Part print with two shaded views. Sizes in mm from the minimum x, y, z corner. Round coordinates to 2 decimals unless told otherwise and drop trailing zeros. Loops run counter-clockwise (first coordinate to the right, second up) from the corner with the lowest first, then second, coordinate; pieces in that order, holes last. Notation, with made-up numbers: (47, -33) -> (105, -33) arc R10 ccw to (105, -27) -> close; hole circle Ø1 at (-39, -34.75). An arc over 180 degrees is marked (long way). Use a Markdown table: item, result. Add a question column.
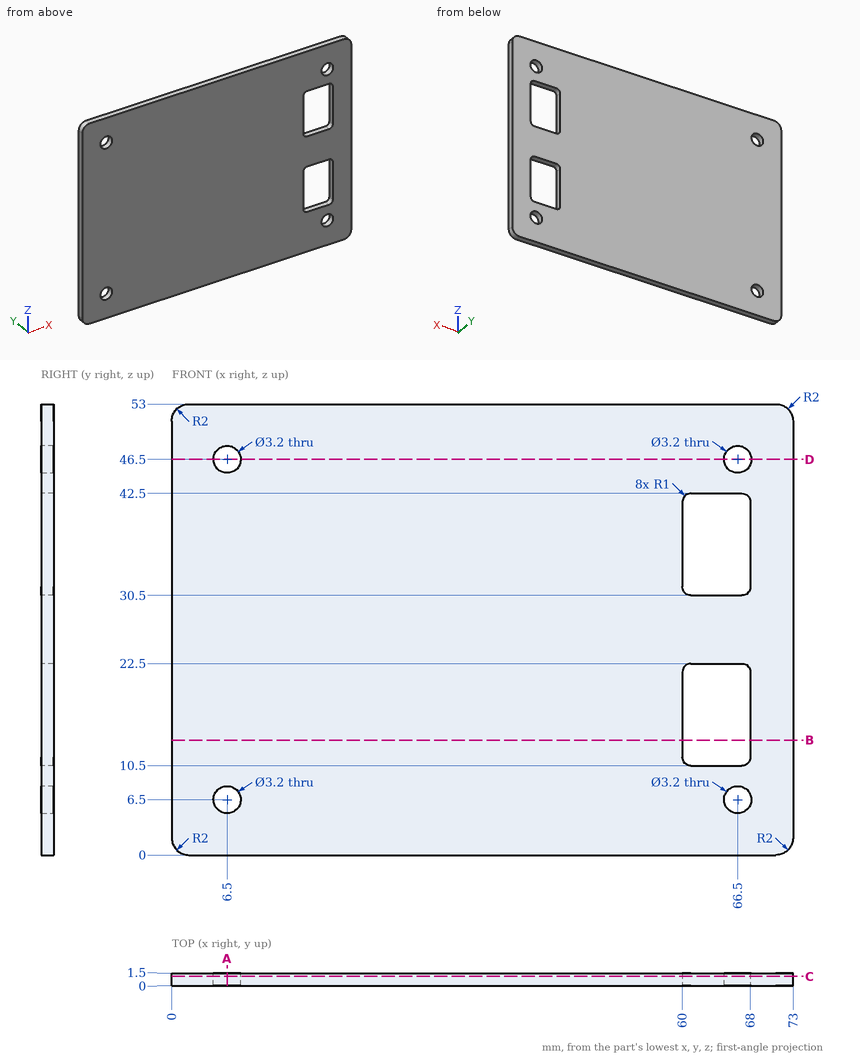
1) Cut at B-B on z = 13.5. Write the cut outline in (x, y), and give its area (3 significant figures).
2) Wall check: probe 1 along Z at (x, y) = (61, 0.65); probe 2 along Z at (x, y) = (66.5, 0.4); probe 3 along X at (y, z) = (0.5, 6.5). Give the ranges that are in metal, low to high. Write a range as from..to.
3) Cut at A-A on x = 6.5. Write the cut outline in (y, z), and give its area (3 significant figures).
4) Cut at C-C on y = 1.1. Write the cut outline in (x, z), and give its area (3 significant figures).
5) Cut at D-D on z = 46.5. Write the cut outline in (x, y).
Established:
| question | item | result |
|---|---|---|
| 1 | outline | (0, 0) -> (60, 0) -> (60, 1.5) -> (0, 1.5) -> close; (68, 0) -> (73, 0) -> (73, 1.5) -> (68, 1.5) -> close |
| 1 | area | 97.5 mm^2 |
| 2 | probe 1 | z = 0..10.5, 22.5..30.5, 42.5..53 |
| 2 | probe 2 | z = 0..4.9, 8.1..10.5, 22.5..30.5, 42.5..44.9, 48.1..53 |
| 2 | probe 3 | x = 0..4.9, 8.1..64.9, 68.1..73 |
| 3 | outline | (0, 0) -> (1.5, 0) -> (1.5, 4.9) -> (0, 4.9) -> close; (0, 8.1) -> (1.5, 8.1) -> (1.5, 44.9) -> (0, 44.9) -> close; (0, 48.1) -> (1.5, 48.1) -> (1.5, 53) -> (0, 53) -> close |
| 3 | area | 69.9 mm^2 |
| 4 | outline | (0, 2) arc R2 ccw to (2, 0) -> (71, 0) arc R2 ccw to (73, 2) -> (73, 51) arc R2 ccw to (71, 53) -> (2, 53) arc R2 ccw to (0, 51) -> close; hole circle Ø3.2 at (6.5, 6.5); hole circle Ø3.2 at (6.5, 46.5); hole (60, 11.5) arc R1 ccw to (61, 10.5) -> (67, 10.5) arc R1 ccw to (68, 11.5) -> (68, 21.5) arc R1 ccw to (67, 22.5) -> (61, 22.5) arc R1 ccw to (60, 21.5) -> close; hole (60, 31.5) arc R1 ccw to (61, 30.5) -> (67, 30.5) arc R1 ccw to (68, 31.5) -> (68, 41.5) arc R1 ccw to (67, 42.5) -> (61, 42.5) arc R1 ccw to (60, 41.5) -> close; hole circle Ø3.2 at (66.5, 6.5); hole circle Ø3.2 at (66.5, 46.5) |
| 4 | area | 3,640 mm^2 |
| 5 | outline | (0, 0) -> (4.9, 0) -> (4.9, 1.5) -> (0, 1.5) -> close; (8.1, 0) -> (64.9, 0) -> (64.9, 1.5) -> (8.1, 1.5) -> close; (68.1, 0) -> (73, 0) -> (73, 1.5) -> (68.1, 1.5) -> close |
